Verification items for the finished model (mm, model axes). Face numbers are marked on the shaded views. A direction names the side the tool comes from. Round coordinates to 2 decimals unless told otherwise and drop trailing zeros. Loops run counter-clockwise (first coordinate to the right, second up) from the corner with the lowest first, then second, coordinate; pieces in that order, holes last.
from build123d import *

# Parameters (mm, degrees)
BOSS_EXTRUDE1_DEPTH = 12.7
SKETCH4_R           = 6.35
CUT_EXTRUDE1_DEPTH  = 7.35
SKETCH5_R           = 9.525
CUT_EXTRUDE2_DEPTH  = 11.43


with BuildPart() as part:
    # Sketch3 → Boss-Extrude1 (new body, symmetric)
    with BuildSketch(Plane(origin=(-49.66137931, -44.143448276, 0), x_dir=(0, 0, 1), z_dir=(-0.747409319, -0.664363839, 0))):
        Polygon((0, 292.094644262), (0, 220.157811167), (14.861770509, 220.157811167), (25.4, 246.581936946), (6.35, 246.581936946), (6.35, 292.094644262), align=None)
    extrude(amount=BOSS_EXTRUDE1_DEPTH, both=True)

    # Sketch4 → Cut-Extrude1 (cut, through all)
    with BuildSketch(Plane.XY.offset(6.35)):
        with Locations((-228.6, 157.1625)):
            Circle(SKETCH4_R)
    extrude(amount=-CUT_EXTRUDE1_DEPTH, mode=Mode.SUBTRACT)

    # Sketch5 → Cut-Extrude2 (cut)
    with BuildSketch(Plane(origin=(-16.673775789, 18.757997763, -62.930465953), x_dir=(0.969242963, 0.07030135, -0.235851222), z_dir=(0.246105828, -0.276869057, 0.928857065))):
        with Locations((-193.99687807, 130.601446216)):
            Circle(SKETCH5_R)
    extrude(amount=-CUT_EXTRUDE2_DEPTH, mode=Mode.SUBTRACT)


solid = part.part
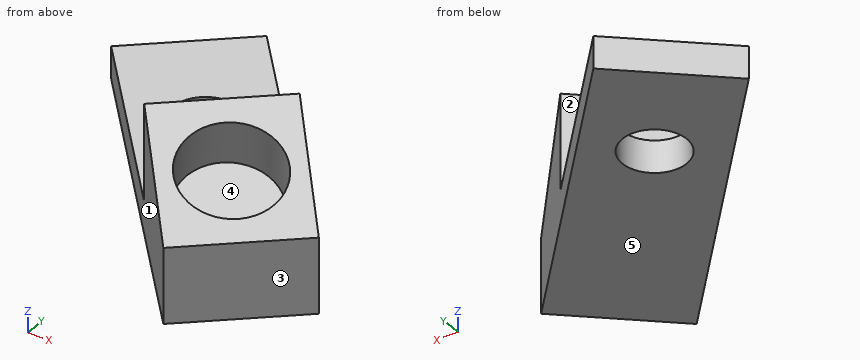
1. Section check A-A (x = -228.6). Enter the section's corners in (y, z), then the cut area to 3 significant figures.
2. Section check C-C (y = 147). Enter the section's corners in (x, z), then the cut area to 3 significant figures.
3. Scan lines: L1, parallel to Y at x = -228.6, z = 4; L2, parallel to Z at x = -240, y = 160; L3, parallel to Y at x = -208, z = 13.5. Record each from-to range of solid material in increasing order.
4. Gauge pin test, flat ends, axial feed: P1, Ø4, axis at x = -215, z = 5, coming from the -Y side; P2, Ø11.5, axis at x = -228.6, y = 157.16, coming from the +Z side; P3, Ø8, axis at y = 124.5, z = 14, coming from the -X side; P4, Ø3, axis at x = -196, z = 18, coming from the +Y side. Record the tip position at first contact, or that the pin passes through.
5. Tool access check on the marked faces 1 and 2. Record the directions out of +Z, -Z, +X, -X, +Y, -Y that give a thin tool (end or side, any length) a straight path to the whole face; none if there is none.
6. Section check D-D (x = -245.5). Enter the section's corners in (y, z).
7. Release check for a two-part mould opening along X. For the marked faces 3, 4 and 5 record: released by +X, released by -X, zero draft, split by the parting line, or undercut.
8. Section check B-B (y = 154.5). Enter the section's corners in (x, z).
Taken from the geometry:
1. outline: (138.05, 0) - (150.81, 0) - (150.81, 6.35) - (138.05, 6.35) - close; (163.51, 0) - (176.28, 0) - (176.28, 6.35) - (163.51, 6.35) - close
1. area: 162 mm2
2. outline: (-236.56, 0) - (-202.57, 0) - (-202.57, 24.55) - (-205.78, 25.4) - (-205.78, 6.35) - (-236.56, 6.35) - close
2. area: 275 mm2
3. L1: y = 138.05 to 150.81, 163.51 to 176.28
3. L2: z = 0 to 6.35
3. L3: y = 114.87 to 122.58, 142.16 to 145.03
4. P1: stops at y = 120.5
4. P2: passes through
4. P3: stops at x = -220.11
4. P4: stops at y = 141.29
5. face 1: +Z, -Z, -X, -Y
5. face 2: +Z, -X, +Y
6. outline: (157.06, 0) - (172.59, 0) - (172.59, 6.35) - (157.06, 6.35) - close
7. face 3: released by +X
7. face 4: undercut
7. face 5: zero draft
8. outline: (-243.23, 0) - (-234.36, 0) - (-234.36, 6.35) - (-243.23, 6.35) - close; (-222.84, 0) - (-209.24, 0) - (-209.24, 6.35) - (-222.84, 6.35) - close
